Geometry: final body of the model. Coordinates: model frame, mm. A direction names the side the tool comes from. Give positions to 0.01 mm unless a question says otherwise; leave off trailing zeros. Loops run counter-clockwise (first coordinate to the right, second up) from the corner with the lowest first, then second, coordinate; pieces in that order, holes last. Notation, with made-up numbers: M -37,38 L 6,38 A21 cw 6,69 Z; hole C 5.25,-16.5 d2. An arc over 180 degrees is marked long. One line per question, with ' | ' between items. Start each with the question number.
from build123d import *

# Parameters (mm, degrees)
F1_DEPTH = 2
F3_DEPTH = 2
F4_R     = 2
F5_DEPTH = 9.46


with BuildPart() as f1:
    # F0 (on Top) → F1 (new body)
    with BuildSketch(Plane.XY):
        with BuildLine():
            Line((-2.95, -4.95), (2.95, -4.95))
            ThreePointArc((2.95, -4.95), (4.364214, -4.364214), (4.95, -2.95))
            Line((4.95, -2.95), (4.95, 2.95))
            ThreePointArc((4.95, 2.95), (4.364214, 4.364214), (2.95, 4.95))
            Line((2.95, 4.95), (-2.95, 4.95))
            ThreePointArc((-2.95, 4.95), (-4.364214, 4.364214), (-4.95, 2.95))
            Line((-4.95, 2.95), (-4.95, -2.95))
            ThreePointArc((-4.95, -2.95), (-4.364214, -4.364214), (-2.95, -4.95))
        make_face()
    extrude(amount=F1_DEPTH)

    # F2 (on face) → F3 (join)
    with BuildSketch(Plane.XY.offset(2)):
        with BuildLine():
            Line((-4, -6), (4, -6))
            ThreePointArc((4, -6), (5.414214, -5.414214), (6, -4))
            Line((6, -4), (6, 4))
            ThreePointArc((6, 4), (5.414214, 5.414214), (4, 6))
            Line((4, 6), (-4, 6))
            ThreePointArc((-4, 6), (-5.414214, 5.414214), (-6, 4))
            Line((-6, 4), (-6, -4))
            ThreePointArc((-6, -4), (-5.414214, -5.414214), (-4, -6))
        make_face()
    extrude(amount=F3_DEPTH)

    # F4 (on face) → F5 (join)
    with BuildSketch(Plane.XY.offset(4)):
        Circle(F4_R)
    extrude(amount=F5_DEPTH)


solid = f1.part
Q1. Contact query for flat-ended pins moving along their axis: pin 1 (2 mm diameter, centred on x = 3.5, y = 4, fed in from +Z); pin 2 (0.6 mm diameter, centred on x = 0.5, z = 1, fed in from -Y); pin 3 (1 mm diameter, centred on y = 1, z = 1, fed in from -X). Output: stop coordinate, or through.
Q2. Material intervals for L1, parallel to X at y = 2.75, z = 1.25; L2, parallel to Z at x = -3.5, y = -1.25; L3, parallel to Z at x = -5.5, y = 1.75, sorted ascending.
Q3. Set-up query: faces 1 (the flat face through (-4.95, 0, 1)), 2 (the flat face through (4.95, 0, 1)), 3 (the flat face through (-0.1, -5.2, 2)), 4 (the flat face through (0, 4.95, 1)), 5 (the cylindrical face through (0, -2, 9)). Return all of +Z, -Z, +X, -X, +Y, -Y with unobstructed straight access to the full face (end or side cutting, diameter ignored); none if empty.
Q4. Section A-A, the plane x = 0. Output: boundary loops of the cut face in (y, z), plus the area to 3 significant figures.
Q5. Section D-D, the plane z = 12.25. Output: boundary loops of the cut face in (x, y), plus the area to 3 significant figures.
Q6. Section C-C, the plane y = -2.75. Output: boundary loops of the cut face in (x, z).
Model answer:
1) pin 1: stops at z = 4 | pin 2: stops at y = -4.95 | pin 3: stops at x = -4.95
2) L1: x = -4.95 to 4.95 | L2: z = 0 to 4 | L3: z = 2 to 4
3) face 1: -Z, -X, +Y, -Y | face 2: -Z, +X, +Y, -Y | face 3: -Z | face 4: -Z, +X, -X, +Y | face 5: +Z
4) outline: M -6,2 L -4.95,2 L -4.95,0 L 4.95,0 L 4.95,2 L 6,2 L 6,4 L 2,4 L 2,13.46 L -2,13.46 L -2,4 L -6,4 Z | area: 81.6 mm^2
5) outline: C 0,0 d4 | area: 12.6 mm^2
6) outline: M -6,2 L -4.95,2 L -4.95,0 L 4.95,0 L 4.95,2 L 6,2 L 6,4 L -6,4 Z
